For this review, take the finished solid that the model builds, in its own axes (mm). Face numbers are marked on the shaded views. A direction names the side the tool comes from. Round coordinates to 2 decimals unless told otherwise and drop trailing zeros. Order: outer loops, then holes, each group sorted by start corner. A loop starts at its lowest first (then second) coordinate and runs counter-clockwise, first axis right, second up. Notation, with made-up numbers: (78.25, 63) - (91.25, 63) arc R27 cw to (91.25, 96) - close; hole circle Ø8 at (12, -19.5). An arc over 180 degrees is marked (long way). One line per question, with ' | ' between items.
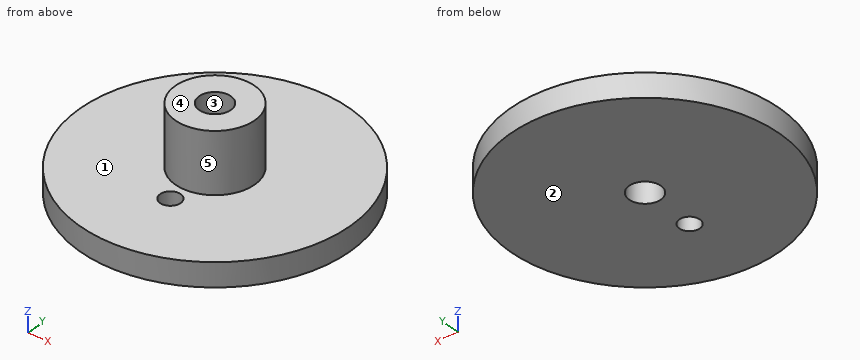
```python
from build123d import *

# Parameters (mm, degrees)
F0_R     = 8.5
F0_R_2   = 1
F1_DEPTH = 1.5
F2_R     = 2.5
F2_R_2   = 1
F3_DEPTH = 3.8
F4_R     = 0.6498381819
F5_DEPTH = 1.5


# Not quite as in the source:
# - a feature names something its author has since deleted; it is built from what else it names


with BuildPart() as f1:
    # F0 (on Top) → F1 (new body)
    with BuildSketch(Plane.XY):
        Circle(F0_R)
        Circle(F0_R_2, mode=Mode.SUBTRACT)
    extrude(amount=F1_DEPTH)

    # F2 (on face) → F3 (join)
    with BuildSketch(Plane.XY.offset(1.5)):
        Circle(F2_R)
        Circle(F2_R_2, mode=Mode.SUBTRACT)
    extrude(amount=F3_DEPTH)

    # F4 (on Top) → F5 (cut, through all)
    with BuildSketch(Plane.XY):
        with Locations((0, -3.5616646055)):
            Circle(F4_R)
    extrude(amount=F5_DEPTH, mode=Mode.SUBTRACT)


solid = f1.part
```
(1) We need section D-D on y = -4. State the section outline as (x, z) points.
Output values:
outline: (-7.5, 0) - (-0.48, 0) - (-0.48, 1.5) - (-7.5, 1.5) - close; (0.48, 0) - (7.5, 0) - (7.5, 1.5) - (0.48, 1.5) - close
(2) We need section A-A on y = 0. State the section outline as (x, z) points.
Output values:
outline: (-8.5, 0) - (-1, 0) - (-1, 5.3) - (-2.5, 5.3) - (-2.5, 1.5) - (-8.5, 1.5) - close; (1, 0) - (8.5, 0) - (8.5, 1.5) - (2.5, 1.5) - (2.5, 5.3) - (1, 5.3) - close
(3) Insertion check: pin 1 (8.5 mm diameter, centred on x = 0, y = -3.5, fed in from +Z); pin 2 (2 mm diameter, centred on x = -2.5, z = 2, fed in from +Y); pin 3 (1 mm diameter, centred on x = 0, y = -3.56, fed in from +Z); pin 4 (1.5 mm diameter, centred on x = 6.5, y = 0.5, fed in from +Z). Each pin has a flat end and moves straight along its axis. Give the tip position at first contact, or say it passes through.
Output values:
pin 1: z = 5.3 | pin 2: y = 8.34 | pin 3: through | pin 4: z = 1.5
(4) We need section C-C on z = 4.05. State the section outline as (x, y) points.
Output values:
outline: circle Ø5 at (0, 0); hole circle Ø2 at (0, 0)
(5) We need section B-B on x = 0. State the section outline as (y, z) points, plus the area to 3 significant figures.
Output values:
outline: (-8.5, 0) - (-4.21, 0) - (-4.21, 1.5) - (-8.5, 1.5) - close; (-2.91, 0) - (-1, 0) - (-1, 5.3) - (-2.5, 5.3) - (-2.5, 1.5) - (-2.91, 1.5) - close; (1, 0) - (8.5, 0) - (8.5, 1.5) - (2.5, 1.5) - (2.5, 5.3) - (1, 5.3) - close | area: 32.0 mm^2
(6) Mouldability with a two-part tool opening along Y and no side actions: class the marked faces 3, 4 and 5 as released by +Y, released by -Y, zero draft, split by the parting line, or undercut.
Output values:
face 3: undercut | face 4: zero draft | face 5: split by the parting line
(7) For the marked faces 1 and 2, list the 3-axis set-ups (+Z, -Z, +X, -X, +Y, -Y) from which the entire face can be reached by the end or side of a thin tool; tool diameter is ignored.
Output values:
face 1: +Z | face 2: -Z, +X, -X, +Y, -Y
(8) For probe 1 along Y at (x, z) = (0, 0.75); probe 2 along Y at (x, z) = (-0.25, 0.3); probe 3 along Y at (x, z) = (0, 4.15), list the stretches that pass through material, from the lowest coordinate up. Write a range as [from, to].
Output values:
probe 1: [-8.5, -4.21], [-2.91, -1], [1, 8.5] | probe 2: [-8.5, -4.16], [-2.96, -0.97], [0.97, 8.5] | probe 3: [-2.5, -1], [1, 2.5]
